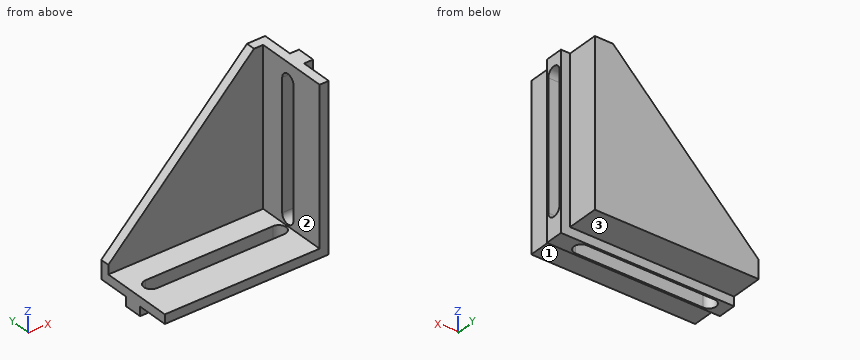
from build123d import *

# Parameters (mm, degrees)
F1_DEPTH  = 45
F3_DEPTH  = 40
F4_W      = 90
F4_H      = 10
F5_DEPTH  = 5
F6_W      = 10
F6_H      = 95
F7_DEPTH  = 5
F9_DEPTH  = 10
F11_DEPTH = 10


with BuildPart() as f1:
    # F0 (on Front) → F1 (new body)
    with BuildSketch(Plane.XZ):
        Polygon((-90, 10), (-90, 0), (0, 0), (0, 90), (-10, 90), align=None)
    extrude(amount=F1_DEPTH)

    # F2 (on face) → F3 (cut)
    with BuildSketch(Plane.XZ.offset(45)):
        Polygon((-10, 90), (-90, 10), (-90, 5), (-5, 5), (-5, 90), align=None)
    extrude(amount=-F3_DEPTH, mode=Mode.SUBTRACT)

    # F4 (on face) → F5 (join)
    with BuildSketch(Plane(origin=(0, 0, 0), x_dir=(1, 0, 0), z_dir=(0, 0, -1))):
        with Locations((-45, 22.5)):
            Rectangle(F4_W, F4_H)
    extrude(amount=F5_DEPTH)

    # F6 (on face) → F7 (join)
    with BuildSketch(Plane.YZ):
        with Locations((-22.5, 42.5)):
            Rectangle(F6_W, F6_H)
    extrude(amount=F7_DEPTH)

    # F8 (on face) → F9 (cut, through all)
    with BuildSketch(Plane.YZ.offset(5)):
        with BuildLine():
            ThreePointArc((-18.5, 80), (-22.5, 84), (-26.5, 80))
            Line((-26.5, 80), (-26.5, 9.960906))
            ThreePointArc((-26.5, 9.960906), (-22.5, 5.999809), (-18.5, 9.960906))
            Line((-18.5, 9.960906), (-18.5, 80))
        make_face()
    extrude(amount=-F9_DEPTH, mode=Mode.SUBTRACT)

    # F10 (on face) → F11 (cut, through all)
    with BuildSketch(Plane(origin=(0, 0, -5), x_dir=(1, 0, 0), z_dir=(0, 0, -1))):
        with BuildLine():
            ThreePointArc((-80, 26.5), (-84, 22.5), (-80, 18.5))
            Line((-80, 18.5), (-10, 18.5))
            ThreePointArc((-10, 18.5), (-6, 22.5), (-10, 26.5))
            Line((-10, 26.5), (-80, 26.5))
        make_face()
    extrude(amount=-F11_DEPTH, mode=Mode.SUBTRACT)


solid = f1.part
Source: CAD feature listing. Evaluate the final solid. Frame: model axes, mm. Face numbers are marked on the shaded views. A direction names the side the tool comes from. Round coordinates to 2 decimals unless told otherwise and drop trailing zeros. Loops run counter-clockwise (first coordinate to the right, second up) from the corner with the lowest first, then second, coordinate; pieces in that order, holes last. Notation, with made-up numbers: M 23,28.5 L 61,28.5 A20 cw 61,64.5 Z; hole C 21,36.5 d4. An arc over 180 degrees is marked long. Return JSON: item names as keys, results as strings. Group by question number.
1. Section query A-A on x = -65.5. Output: boundary loops of the cut face in (y, z).
2. Section query C-C on y = -21. Output: boundary loops of the cut face in (x, z), and give its area (3 significant figures).
3. Material intervals for line 1 along Y through (x, z) = (1.5, 60); line 2 along Y through (x, z) = (-15, 13.5), sorted ascending. Write a range as from..to.
4. Pin query (flat end, axial travel): pin 1 (4 mm diameter, centred on y = -37, z = 65.5, fed in from +X); pin 2 (5 mm diameter, centred on x = -45, y = -12, fed in from +Z); pin 3 (12 mm diameter, centred on x = -35, y = -8, fed in from +Z). Return the tip coordinate at first contact, or that it passes through.
5. Section query B-B on z = 55. Output: boundary loops of the cut face in (x, y), and give its area (3 significant figures).
6. Section query D-D on y = -36.5. Output: boundary loops of the cut face in (x, z).
7. Reachability of the marked faces 1, 2 and 3 from +Z, -Z, +X, -X, +Y, -Y: full face, straight path, thin tool, end or side. Return the list, or none.
Checks:
{
 "1": {"outline": "M -45,0 L -27.5,0 L -27.5,-5 L -26.5,-5 L -26.5,5 L -45,5 Z; M -18.5,-5 L -17.5,-5 L -17.5,0 L 0,0 L 0,34.5 L -5,34.5 L -5,5 L -18.5,5 Z"},
 "2": {"outline": "M -90,-5 L -83.71,-5 L -83.71,5 L -90,5 Z; M -6.29,-5 L 5,-5 L 5,6.29 L -5,6.29 L -5,5 L -6.29,5 Z; M -5,83.71 L 5,83.71 L 5,90 L -5,90 Z", "area": "252 mm²"},
 "3": {"line 1": "y = -27.5..-26.5, -18.5..-17.5", "line 2": "y = -5..0"},
 "4": {"pin 1": "stops at x = 0", "pin 2": "stops at z = 5", "pin 3": "stops at z = 70.2"},
 "5": {"outline": "M -45,-5 L -5,-5 L -5,-18.5 L 5,-18.5 L 5,-17.5 L 0,-17.5 L 0,0 L -45,0 Z; M -5,-45 L 0,-45 L 0,-27.5 L 5,-27.5 L 5,-26.5 L -5,-26.5 Z", "area": "395 mm²"},
 "6": {"outline": "M -90,0 L 0,0 L 0,90 L -5,90 L -5,5 L -90,5 Z"},
 "7": {"face 1": "-Z, +X, -X, -Y", "face 2": "+Z, -X, -Y", "face 3": "-Z, +X, -X, +Y"}
}
